from build123d import *

# Parameters (mm, degrees)
CROQUIS1_W              = 440.5
CROQUIS1_H              = 120
CROQUIS1_R              = 1.55
SALIENTE_EXTRUIR1_DEPTH = 2
CROQUIS2_W              = 440.5
CROQUIS2_H              = 120
CROQUIS2_W_2            = 439.5
CROQUIS2_H_2            = 119
CORTAR_EXTRUIR1_DEPTH   = 2
CORTAR_EXTRUIR2_DEPTH   = 2
REDONDEO1_R             = 1


with BuildPart() as part:
    # Croquis1 → Saliente-Extruir1 (new body)
    with BuildSketch(Plane(origin=(0, 0, 0), x_dir=(1, 0, 0), z_dir=(0, 1, 0))):
        with Locations((220.25, 60)):
            Rectangle(CROQUIS1_W, CROQUIS1_H)
        with Locations(Location((12.5, 15, 0), (0, 0, 270))):
            Circle(CROQUIS1_R, mode=Mode.SUBTRACT)
        with Locations(Location((12.5, 110, 0), (0, 0, 270))):
            Circle(CROQUIS1_R, mode=Mode.SUBTRACT)
        with Locations(Location((428, 15, 0), (0, 0, 90))):
            Circle(CROQUIS1_R, mode=Mode.SUBTRACT)
        with Locations(Location((428, 110, 0), (0, 0, 90))):
            Circle(CROQUIS1_R, mode=Mode.SUBTRACT)
    extrude(amount=SALIENTE_EXTRUIR1_DEPTH)

    # Croquis2 → Cortar-Extruir1 (cut)
    with BuildSketch(Plane.XZ):
        with Locations((220.25, -60)):
            Rectangle(CROQUIS2_W, CROQUIS2_H)
        with Locations((220.25, -60)):
            Rectangle(CROQUIS2_W_2, CROQUIS2_H_2, mode=Mode.SUBTRACT)
    extrude(amount=-CORTAR_EXTRUIR1_DEPTH, mode=Mode.SUBTRACT)

    # Croquis3 → Cortar-Extruir2 (cut)
    with BuildSketch(Plane.XZ):
        Polygon((85.5, -119.5), (119.5, -119.5), (119.5, -113.5), (108.5, -113.5), (108.5, -96.5), (96.5, -96.5), (96.5, -113.5), (85.5, -113.5), align=None)
    extrude(amount=-CORTAR_EXTRUIR2_DEPTH, mode=Mode.SUBTRACT)

    # Redondeo1
    redondeo1_edges = [part.edges().sort_by_distance(p)[0] for p in [
        (85.5, 1, -113.5),
        (96.5, 1, -113.5),
        (96.5, 1, -96.5),
        (108.5, 1, -96.5),
        (108.5, 1, -113.5),
        (119.5, 1, -113.5),
    ]]
    fillet(redondeo1_edges, radius=REDONDEO1_R)


solid = part.part
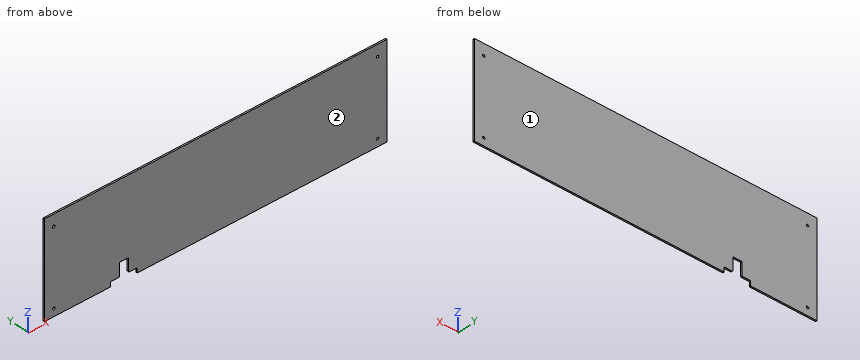
Geometry check sheet. Reference: the model listing, model coordinates, mm. Face numbers are marked on the shaded views. Round coordinates to 2 decimals unless told otherwise and drop trailing zeros. One line per item, written item: value. Start each with the question number.
(1) Go/stop test with flat-tipped pins: pin 1 Ø0.6 at (x, y) = (93, 1.5) entering from -Z; pin 2 Ø0.6 at (x, y) = (101.5, 1) entering from -Z. Record where each tip stops, or that it passes through.
(2) Scan lines: line 1 (X direction, y = 0.9, z = -110); line 2 (X direction, y = 1.4, z = -15); line 3 (X direction, y = 1.05, z = -101). Record each from-to range of solid material in increasing order. Write a range as [from, to].
(3) Draft check along Y on the marked faces 1 and 2. Enter one of: +Y half, -Y half, draft (parallel to the pull), parting line (faces both ways), or undercut.
Answer:
1. pin 1: z = -113.5
1. pin 2: z = -96.5
2. line 1: [0.5, 10.95], [14.05, 96.5], [108.5, 426.45], [429.55, 440]
2. line 2: [0.5, 10.95], [14.05, 426.45], [429.55, 440]
2. line 3: [0.5, 96.5], [108.5, 440]
3. face 1: +Y half
3. face 2: -Y half
